Geometry check sheet. Reference: the model listing, model coordinates, mm. A direction names the side the tool comes from. Round coordinates to 2 decimals unless told otherwise and drop trailing zeros. Loops run counter-clockwise (first coordinate to the right, second up) from the corner with the lowest first, then second, coordinate; pieces in that order, holes last. Notation, with made-up numbers: (10, 79) -> (26, 79) arc R27 ccw to (26, 110) -> close; hole circle Ø1 at (14, 38). An arc over 180 degrees is marked (long way). Use one line per item in the form item = value.
from build123d import *

# Parameters (mm, degrees)
ESQUISSE1_R             = 10.5
BOSS_EXTRU_1_DEPTH      = 4
ESQUISSE2_R             = 13
BOSS_EXTRU_2_DEPTH      = 2
ESQUISSE3_R             = 1.5
ENL_V_MAT_EXTRU_1_DEPTH = 20.339079606


with BuildPart() as part:
    # Esquisse1 → Boss.-Extru.1 (new body)
    with BuildSketch(Plane(origin=(0, 0, 0), x_dir=(1, 0, 0), z_dir=(0, 1, 0))):
        with Locations(Location((0, 0, 0), (0, 0, 270))):
            Circle(ESQUISSE1_R)
    extrude(amount=BOSS_EXTRU_1_DEPTH)

    # Esquisse2 → Boss.-Extru.2 (add)
    with BuildSketch(Plane.XZ):
        with Locations(Location((0, 0, 0), (0, 0, 270))):
            Circle(ESQUISSE2_R)
    extrude(amount=BOSS_EXTRU_2_DEPTH)

    # Esquisse3 → Enlèv. mat.-Extru.1 (cut, through all)
    with BuildSketch(Plane(origin=(0, 4, 0), x_dir=(1, 0, 0), z_dir=(0, 1, 0))):
        with Locations(Location((-7.999447207, -0.094044544, 0), (0, 0, 270))):
            Circle(ESQUISSE3_R)
        with Locations(Location((-0.094044544, 7.999447207, 0), (0, 0, 270))):
            Circle(ESQUISSE3_R)
        with Locations(Location((0.094044544, -7.999447207, 0), (0, 0, 270))):
            Circle(ESQUISSE3_R)
        with Locations(Location((7.999447207, 0.094044544, 0), (0, 0, 270))):
            Circle(ESQUISSE3_R)
    extrude(amount=-ENL_V_MAT_EXTRU_1_DEPTH, mode=Mode.SUBTRACT)


solid = part.part
1. Gauge pin test, flat ends, axial feed: pin 1 (5 mm diameter, centred on x = -8, z = 0.09, fed in from +Y); pin 2 (3 mm diameter, centred on y = 2.5, z = -4, fed in from -X); pin 3 (2 mm diameter, centred on x = 7, y = -0.5, fed in from +Z). Record the tip position at first contact, or that the pin passes through.
Return value:
pin_1 = 4
pin_2 = -10.2
pin_3 = 11.53
2. Section check C-C (y = 2.2). Record the boundary of the cut face in (x, z).
Return value:
outline = circle Ø21 at (0, 0); hole circle Ø3 at (-8, 0.09); hole circle Ø3 at (-0.09, -8); hole circle Ø3 at (0.09, 8); hole circle Ø3 at (8, -0.09)
3. Tool access check on faces 1 (the cylindrical face through (-9.464, 1.042, -0.231)), 2 (the flat face through (6, 0, 9)). Record the directions out of +Z, -Z, +X, -X, +Y, -Y that give a thin tool (end or side, any length) a straight path to the whole face; none if there is none.
Return value:
face_1 = +Y, -Y
face_2 = +Y
4. Section check A-A (z = 0.5). Record the boundary of the cut face in (x, y).
Return value:
outline = (-12.99, -2) -> (-9.44, -2) -> (-9.44, 4) -> (-10.49, 4) -> (-10.49, 0) -> (-12.99, 0) -> close; (-6.56, -2) -> (6.62, -2) -> (6.62, 4) -> (-6.56, 4) -> close; (9.38, -2) -> (12.99, -2) -> (12.99, 0) -> (10.49, 0) -> (10.49, 4) -> (9.38, 4) -> close
5. Section check D-D (x = -2.5). Record the boundary of the cut face in (y, z).
Return value:
outline = (-2, -12.76) -> (0, -12.76) -> (0, -10.2) -> (4, -10.2) -> (4, 10.2) -> (0, 10.2) -> (0, 12.76) -> (-2, 12.76) -> close
6. Material ranges on line 1 along Y through (x, z) = (8, -8.5); line 2 along X through (y, z) = (1.75, 8.5); line 3 along X through (y, z) = (-0.75, -7.25), recorded low to high.
Return value:
line_1 = -2 to 0
line_2 = -6.16 to -1.32, 1.51 to 6.16
line_3 = -10.79 to -1.39, 1.21 to 10.79
7. Section check B-B (x = -5.5). Record the boundary of the cut face in (y, z), then the cut area to 3 significant figures.
Return value:
outline = (-2, -11.78) -> (0, -11.78) -> (0, -8.94) -> (4, -8.94) -> (4, 8.94) -> (0, 8.94) -> (0, 11.78) -> (-2, 11.78) -> close
area = 119 mm2
8. Mould release check, pull along Z, two halves, no side actions. Record for faces 3 (the cylindrical face through (-0.03, 1.04, -9.5)), 4 (the flat face through (0, -2, 0)), 5 (the cylindrical face through (-7.91, -0.986, 10.316)): released by +Z, released by -Z, zero draft, split by the parting line, or undercut.
Return value:
face_3 = undercut
face_4 = zero draft
face_5 = split by the parting line
